Study the drawing (mm; zero at the part's minimum x, y, z) and answer. A direction names the side the tool comes from. Round coordinates to 2 decimals unless told otherwise and drop trailing zeros. Loops run counter-clockwise (first coordinate to the right, second up) from the corner with the lowest first, then second, coordinate; pieces in that order, holes last. Notation, with made-up numbers: (79.5, -9.75) - (103.5, -9.75) arc R4 cw to (103.5, -5.75) - close; hole circle Ø4 at (9.5, 45.25). An arc over 180 degrees is marked (long way). One line per item, written item: value.
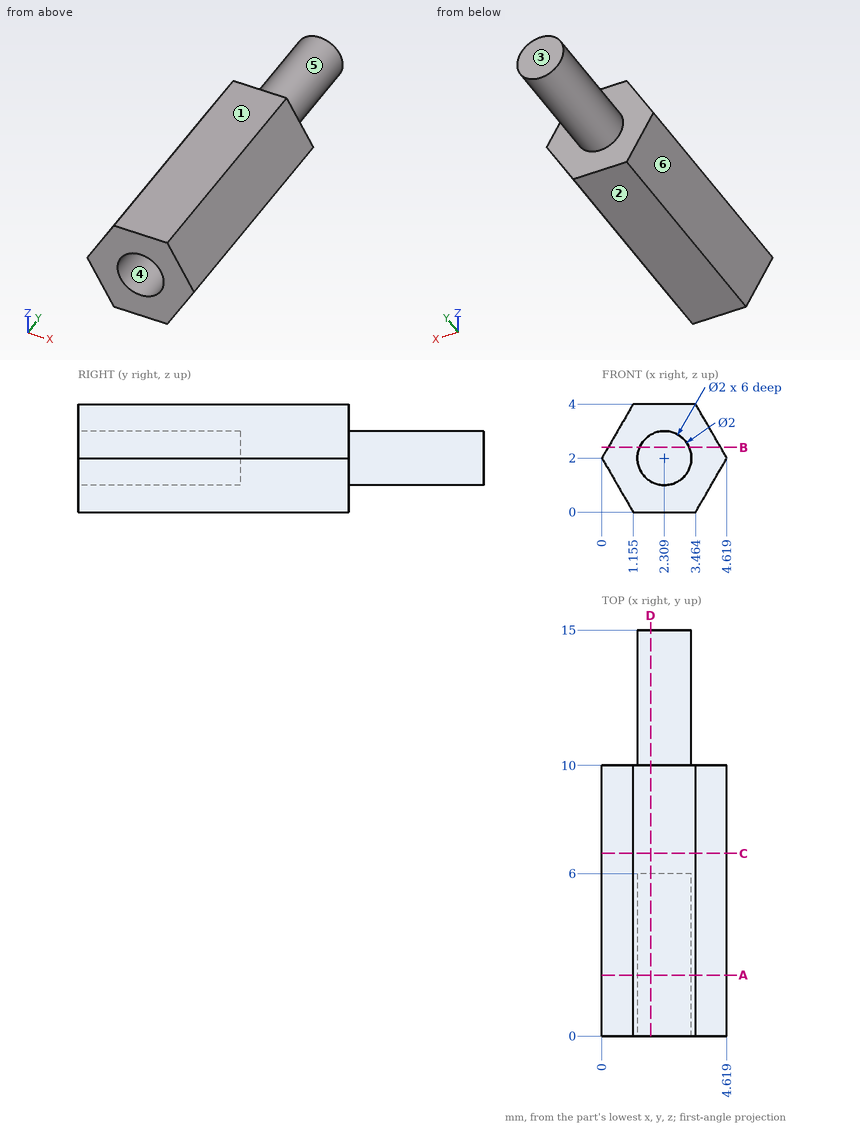
1) A cutting plane is placed at C-C on y = 6.75. Give the vertices of the cut face in (x, z) (1 decimal).
Final values:
outline: (0, 2) - (1.2, 0) - (3.5, 0) - (4.6, 2) - (3.5, 4) - (1.2, 4) - close
2) For the marked faces 5 and 6, determine the directions among +Z, -Z, +X, -X, +Y, -Y from which every point of the face is accessible in a straight line to the end or side of a thin tool.
Final values:
face 5: +Y
face 6: -Z, -X, +Y, -Y
3) A cutting plane is placed at A-A on y = 2.25. Give the vertices of the cut face in (x, z) (1 decimal), and give its area (3 significant figures).
Final values:
outline: (0, 2) - (1.2, 0) - (3.5, 0) - (4.6, 2) - (3.5, 4) - (1.2, 4) - close; hole circle Ø2 at (2.3, 2)
area: 10.7 mm2
4) A cutting plane is placed at B-B on z = 2.4. Give the vertices of the cut face in (x, y).
Final values:
outline: (0.23, 0) - (1.39, 0) - (1.39, 6) - (3.23, 6) - (3.23, 0) - (4.39, 0) - (4.39, 10) - (3.23, 10) - (3.23, 15) - (1.39, 15) - (1.39, 10) - (0.23, 10) - close
5) Each of these flat-tipped pins is pushed along its axis until it touches: pin 1 Ø1.2 at (x, z) = (2.31, 2) entering from -Y; pin 2 Ø1 at (x, y) = (2, 13) entering from +Z; pin 3 Ø1 at (y, z) = (6.5, 1) entering from -X. Where does it stop, or does it pass through?
Final values:
pin 1: y = 6
pin 2: z = 3
pin 3: x = 0.29
6) A cutting plane is placed at D-D on x = 1.8. Give the vertices of the cut face in (y, z).
Final values:
outline: (0, 0) - (10, 0) - (10, 1.14) - (15, 1.14) - (15, 2.86) - (10, 2.86) - (10, 4) - (0, 4) - (0, 2.86) - (6, 2.86) - (6, 1.14) - (0, 1.14) - close
7) For a pull along Z with two mould halves and no side action, classify the marked faces 1, 2, 3 and 4 as released by +Z, released by -Z, zero draft, split by the parting line, or undercut.
Final values:
face 1: released by +Z
face 2: released by -Z
face 3: zero draft
face 4: undercut
8) Consider L1, parallel to X at y = 5, z = 1.5 (1 decimal); L2, parallel to Y at x = 2.05, z = 2.5; L3, parallel to X at y = 5.25, z = 2.4 (1 decimal). Determine where each line is inside the solid, lowest interval first.
Final values:
L1: 0.3 to 1.4, 3.2 to 4.3
L2: 6 to 15
L3: 0.2 to 1.4, 3.2 to 4.4
